Source: CAD feature listing. Evaluate the final solid. Frame: model axes, mm. Coordinates: 2 decimals unless noted, no trailing zeros. Loops run counter-clockwise (first coordinate to the right, second up) from the corner with the lowest first, then second, coordinate; pieces in that order, holes last. Notation, with made-up numbers: M 29,87.25 L 68,87.25 A25 ccw 68,115.25 Z; hole C -31.75,48 d2. An arc over 180 degrees is marked long. One line per question, with ' | ' between items. Start each with the question number.
1. Section query D-D, the plane y = 25.3. Output: boundary loops of the cut face in (x, z).
2. Section query C-C, the plane x = -115. Output: boundary loops of the cut face in (y, z), and give its area (3 significant figures).
3. Section query B-B, the plane z = -213. Output: boundary loops of the cut face in (x, y).
4. Mould query, pull axis X, two halves, no side actions, for faces 1 (the cylindrical face through (21.57, 24.99, -64.09)), 2 (the cylindrical face through (-109.59, 24.99, -98.19)), 3 (the cylindrical face through (-114.431, 24.989, -204.632)). Classes: pulls with the +X half, pulls with the -X half, needs draft (parallel to the pull), parting line crosses it, or undercut.
5. Pin query (flat end, axial travel): P1, Ø1, axis at y = 25, z = -178, coming from the -X side. Return the tip coordinate at first contact, or that it passes through.
6. Section query A-A, the plane x = -25.5. Output: boundary loops of the cut face in (y, z), and give its area (3 significant figures).
7. Ray query, probe 1 along Z at (x, y) = (-100, 26.15); probe 2 along Z at (x, y) = (-43.5, 23.7); probe 3 along X at (y, z) = (24.45, -102). Return the intervals inside material, ascending.
Autodesk Inventor part; units mm, degrees
ref_plane "YZ Plane" through (0, 0, 0) normal (1, 0, 0) x (0, 1, 0)
ref_plane "XZ Plane" through (0, 0, 0) normal (0, 1, 0) x (-1, 0, 0)
ref_plane "XY Plane" through (0, 0, 0) normal (0, 0, 1) x (1, 0, 0)
ref_plane "Work Plane1" through (-51.7969, 23.5104, -145.9222) normal (0, 1, 0) x (-1, 0, 0)
sketch "Sketch1" plane through (-51.7969, 23.5104, -145.9222) normal (0, 1, 0) x (-1, 0, 0)
  circle A0 centre (64.1421, 42.8631) radius 8
  circle A1 centre (0, -8.3092) radius 65.3144
  line L0 (80.3944, -8.3092) -> (80.3944, 77.2593)
  arc A2 (68.9502, 88.7036) -> (80.3944, 77.2593) centre (87.3944, 95.7036) ccw
  line L1 (68.9502, 88.7036) -> (-68.9502, 88.7036)
  arc A3 (-80.3944, 77.2593) -> (-68.9502, 88.7036) centre (-87.3944, 95.7036) ccw
  line L2 (-80.3944, 77.2593) -> (-80.3944, -8.3092)
  arc A4 (-80.3944, -8.3092) -> (-15.6866, -87.1584) centre (0, -8.3092) ccw
  arc A5 (15.6866, -87.1584) -> (-15.6866, -87.1584) centre (0, -96.4205) ccw
  arc A6 (15.6866, -87.1584) -> (80.3944, -8.3092) centre (0, -8.3092) ccw
  point P0 (-51.7969, 145.9222)
extrude "Extrusion1" add sketch "Sketch1" along normal blind 3
properties part number "pcb"
Taken from the geometry:
1) outline: M -132.19,-154.23 A80.39 ccw -67.48,-233.08 A18.22 cw -36.11,-233.08 A80.39 ccw 28.6,-154.23 L 28.6,-68.66 A19.73 cw 17.15,-57.22 L -120.75,-57.22 A19.73 cw -132.19,-68.66 Z; hole C -115.94,-103.06 d16; hole C -51.8,-154.23 d130.63
2) outline: M 23.51,-203.92 L 26.51,-203.92 L 26.51,-170.7 L 23.51,-170.7 Z; M 23.51,-137.76 L 26.51,-137.76 L 26.51,-111 L 23.51,-111 Z; M 23.51,-95.11 L 26.51,-95.11 L 26.51,-57.22 L 23.51,-57.22 Z | area: 294 mm^2
3) outline: M -106.66,23.51 L -80.3,23.51 L -80.3,26.51 L -106.66,26.51 Z; M -23.3,23.51 L 3.06,23.51 L 3.06,26.51 L -23.3,26.51 Z
4) face 1: pulls with the +X half | face 2: undercut | face 3: pulls with the -X half
5) P1: x = -128.75
6) outline: M 23.51,-230.2 L 26.51,-230.2 L 26.51,-214.02 L 23.51,-214.02 Z; M 23.51,-94.44 L 26.51,-94.44 L 26.51,-57.22 L 23.51,-57.22 Z | area: 160 mm^2
7) probe 1: -218.57 to -198.3, -110.16 to -57.22 | probe 2: -226.12 to -219.02, -89.45 to -57.22 | probe 3: -132.19 to -123.87, -108.01 to -91.01, -12.58 to 28.6
